Can you work these out from the model? Positions are in its coordinate system, mm. Face numbers are marked on the shaded views. A direction names the side the tool comes from. Coordinates: 2 decimals unless noted, no trailing zeros. Order: outer loops, then holes, each group sorted by start corner. A loop starts at its lowest first (then second) coordinate and runs counter-clockwise, first axis right, second up. Notation, with made-up numbers: (36.25, 17) -> (74.25, 17) arc R21 cw to (74.25, 46) -> close; hole circle Ø9 at (7.25, -14.5). An arc over 180 degrees is marked (long way). Answer as CSV lines item,"result".
from build123d import *

# Parameters (mm, degrees)
F1_DEPTH = 63.5
F0_W     = 25.4
F0_H     = 19.05
F2_DEPTH = 25.4
F3_DEPTH = 7.9375
F4_R     = 6.35


with BuildPart() as f1:
    # F0 (on Front) → F1 (new body, symmetric)
    with BuildSketch(Plane.XZ):
        Polygon((22.225, 9.525), (-41.275, 9.525), (-41.275, -9.525), (41.275, -9.525), (41.275, 9.525), align=None)
    extrude(amount=F1_DEPTH, both=True)

    # F0 (on Front) → F2 (join, symmetric)
    with BuildSketch(Plane.XZ):
        with BuildLine():
            Line((22.225, 27.0002), (22.225, 9.525))
            Line((22.225, 9.525), (41.275, 9.525))
            Line((41.275, 9.525), (41.275, 27.0002))
            ThreePointArc((41.275, 27.0002), (45.9246798487, 38.2255201513), (57.15, 42.8752))
            Line((57.15, 42.8752), (60.325, 42.8752))
            Line((60.325, 42.8752), (60.325, 61.9252))
            Line((60.325, 61.9252), (57.15, 61.9252))
            add(Edge.make_bspline(
                [(53.5478773924, 61.7389440435), (54.7236223027, 61.8188750889), (55.923949642, 61.8811762152), (57.15, 61.9252)],
                knots=[108.7572829366, 108.7572829366, 108.7572829366, 108.7572829366, 111.5045361635, 111.5045361635, 111.5045361635, 111.5045361635], degree=3))
            ThreePointArc((53.5478773924, 61.7389440435), (31.2119993343, 50.3877126182), (22.225, 27.0002))
        make_face()
        with Locations((73.025, 52.4002)):
            Rectangle(F0_W, F0_H)
    extrude(amount=F2_DEPTH, both=True)

    # F0 (on Front) → F3 (join, symmetric)
    with BuildSketch(Plane.XZ):
        with BuildLine():
            add(Edge.make_bspline(
                [(-41.275, 9.525), (-1.0169351027, 27.7810963439), (7.0029063578, 58.5746622675), (53.5478773924, 61.7389440435)],
                knots=[0, 0, 0, 0, 108.7572829366, 108.7572829366, 108.7572829366, 108.7572829366], degree=3))
            Line((-41.275, 9.525), (22.225, 9.525))
            Line((22.225, 9.525), (22.225, 27.0002))
            ThreePointArc((22.225, 27.0002), (31.2119993343, 50.3877126182), (53.5478773924, 61.7389440435))
        make_face()
    extrude(amount=F3_DEPTH, both=True)

    # F4
    f4_edges = [f1.edges().sort_by_distance(p)[0] for p in [
        (-41.275, -63.5, 0),
        (41.275, -63.5, 0),
        (41.275, 63.5, 0),
        (-41.275, 63.5, 0),
    ]]
    fillet(f4_edges, radius=F4_R)

    # F0 (on Front) → F5 (revolve)
    with BuildSketch(Plane.XZ):
        Polygon((85.725, 66.675), (85.725, 61.9252), (85.725, 42.8752), (85.725, 38.1), (111.125, 38.1), (111.125, 66.675), align=None)
    revolve(axis=Axis((85.725, 0, 52.3875), (0, 0, 1)))


solid = f1.part
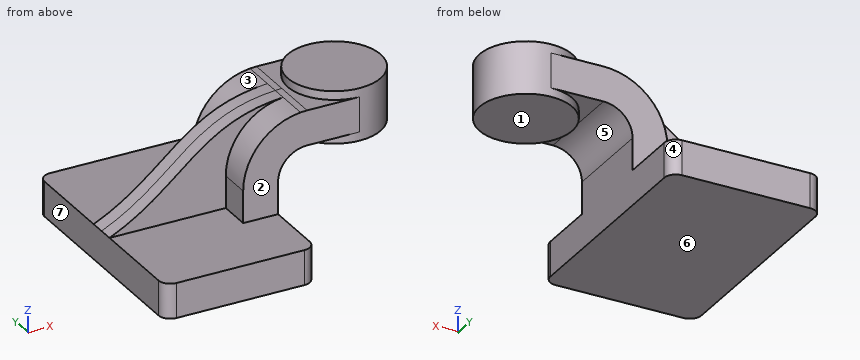
Q1. For P1, Ø10, axis at y = 20, z = 27, coming from the -X side (3 decimals); P2, Ø14.5, axis at x = 65.5, y = -7.5, coming from the -Z side; P3, Ø11, axis at y = 23.5, z = 10, coming from the +X side (3 decimals), each with a flat end and sliding along its axis, tell me the tip position at first contact or that it passes through.
Solution:
P1,"x = 22.225"
P2,"z = 38.1"
P3,"x = 41.275"
Q2. If I drill on line 1 (Y direction, x = 62.5, z = 60); line 2 (X direction, y = 0, z = 9) (3 decimals); line 3 (Z direction, x = 58, y = 14.5), over which ranges is the centre line in solid material (lowest first)?
Solution:
line 1,"-25.4 to 25.4"
line 2,"-41.275 to 41.275"
line 3,"42.88 to 61.93"
Q3. We'd pull the mould along X, two halves only. Please class the marked faces 4, 5, 6 and 7: pulls with the +X half, pulls with the -X half, needs draft (parallel to the pull), parting line crosses it, or undercut.
Solution:
face 4,"pulls with the +X half"
face 5,"undercut"
face 6,"needs draft"
face 7,"pulls with the -X half"
Q4. Which directions (+Z, -Z, +X, -X, +Y, -Y) give clear straight access to the entire face, cutting with the end or side of a thin tool? Please do the marked faces 1, 2 and 3.
Solution:
face 1,"-Z, +X, +Y, -Y"
face 2,"+Z, +X, -X, -Y"
face 3,"+Z, -X, +Y"
Q5. Imagine slicing it at B-B (y = 41.5). List the corners of the cut face in (x, z) for me (3 decimals).
Solution:
outline,"(-41.275, -9.525) -> (41.275, -9.525) -> (41.275, 9.525) -> (-41.275, 9.525) -> close"
Q6. Imagine slicing it at A-A (z = -2). List the corners of the cut face in (x, y) for me (3 decimals), and give its area (3 significant figures).
Solution:
outline,"(-41.275, -57.15) arc R6.35 ccw to (-34.925, -63.5) -> (34.925, -63.5) arc R6.35 ccw to (41.275, -57.15) -> (41.275, 57.15) arc R6.35 ccw to (34.925, 63.5) -> (-34.925, 63.5) arc R6.35 ccw to (-41.275, 57.15) -> close"
area,"10,400 mm2"
